Can you work these out from the drawing? Everything is in mm from the part's minimum corner. Give positions to 0.01 mm unless a question says otherwise; leave off trailing zeros. Order: outer loops, then holes, each group sorted by start corner. A loop starts at its lowest first (then second) coordinate and runs counter-clockwise, first axis right, second up. Notation, with made-up numbers: M 50,83 L 106,83 A36 ccw 106,118 Z; hole C 3,45.25 d8. An arc over 180 degrees is marked long. Answer in a Markdown table with one row per item. Add a question column.
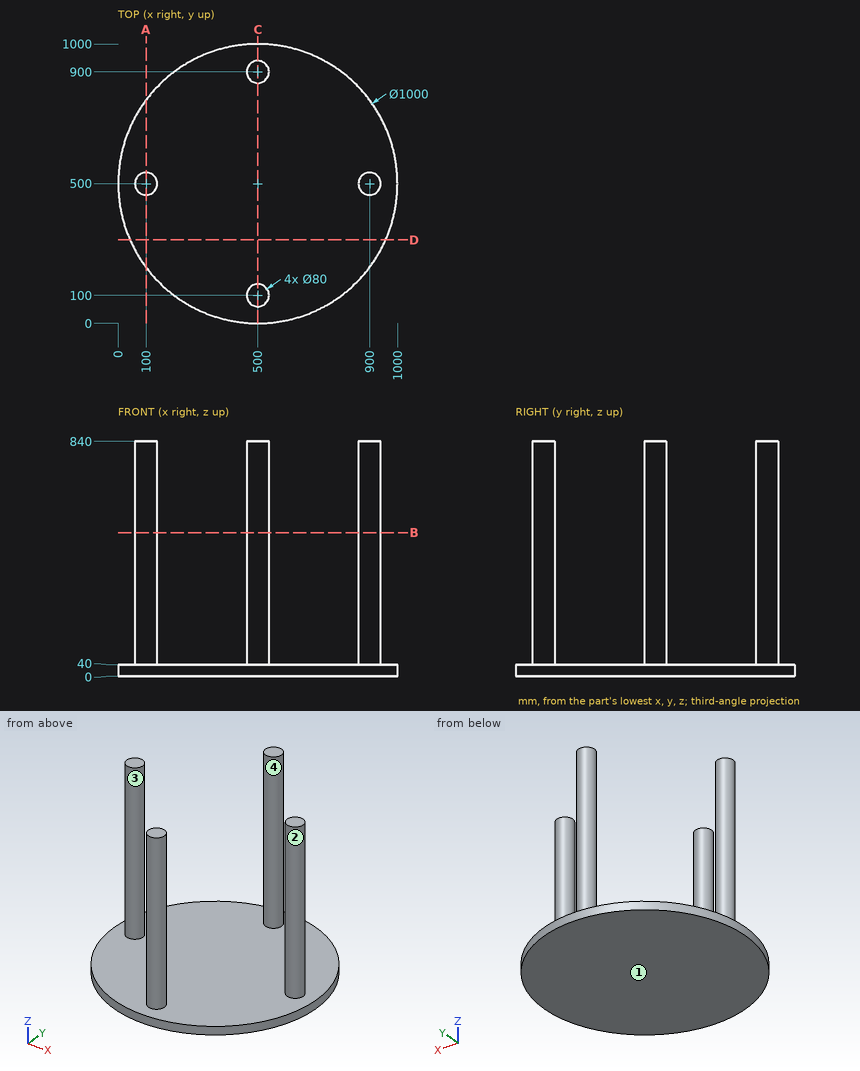
1. Will these pins go through, and if not, where does the flat tip stop? P1, Ø4, axis at x = 303.5, y = 282.5, coming from the +Z side; P2, Ø1, axis at x = 889, z = 604, coming from the -Y side; P3, Ø1.5, axis at x = 506, z = 280.5, coming from the -Y side.
2. Suppose I cut it at C-C on x = 500. List the corners of the cut face in (y, z) for me.
3. Thinking about a two-plate mould opening in X: for the marked faces 1, 2, 3 and 4, which applies, pulls with the +X half, pulls with the -X half, needs draft (parallel to the pull), parting line crosses it, or undercut?
4. Suppose I cut it at A-A on x = 100. List the corners of the cut face in (y, z) for me.
5. Suppose I cut it at D-D on y = 299. List the corners of the cut face in (x, z) for me, plus the area to 3 significant figures.
6. Suppose I cut it at B-B on z = 513. List the corners of the cut face in (x, y) for me.
7. If I drill on line 1 along Z through (x, y) = (172, 854); line 2 along Y through (x, z) = (527, 53); line 3 along X through (y, z) = (483.5, 624.5), over which ranges is the centre line in solid material (lowest first)? Write a range as [from, to].
Findings below:
| question | item | result |
|---|---|---|
| 1 | P1 | z = 40 |
| 1 | P2 | y = 461.4 |
| 1 | P3 | y = 60.35 |
| 2 | outline | M 0,0 L 1000,0 L 1000,40 L 940,40 L 940,840 L 860,840 L 860,40 L 140,40 L 140,840 L 60,840 L 60,40 L 0,40 Z |
| 3 | face 1 | needs draft |
| 3 | face 2 | undercut |
| 3 | face 3 | undercut |
| 3 | face 4 | parting line crosses it |
| 4 | outline | M 200,0 L 800,0 L 800,40 L 540,40 L 540,840 L 460,840 L 460,40 L 200,40 Z |
| 5 | outline | M 42.18,0 L 957.82,0 L 957.82,40 L 42.18,40 Z |
| 5 | area | 36,600 mm2 |
| 6 | outline | C 100,500 d80; C 500,100 d80; C 500,900 d80; C 900,500 d80 |
| 7 | line 1 | [0, 40] |
| 7 | line 2 | [70.49, 129.51], [870.49, 929.51] |
| 7 | line 3 | [63.56, 136.44], [863.56, 936.44] |
